Design review of the part built by this model. Coordinates are the model's own, in mm. A direction names the side the tool comes from. Coordinates: 2 decimals unless noted, no trailing zeros. Write each loop counter-clockwise with the first axis right and the second up, starting at its lowest first coordinate (ties: lowest second). Pieces come first, ordered by that corner, then holes. Notation, with made-up numbers: M 58,57.5 L 87,57.5 A26 ccw 87,93.5 Z; hole C 32.5,31 d10. An arc over 180 degrees is marked long. Return JSON: item names as keys, results as strings. Group by question number.
```python
from build123d import *

# Parameters (mm, degrees)
F0_W     = 254
F0_H     = 88.9
F0_R     = 3.81
F0_R_2   = 3.937
F1_DEPTH = 127
F2_T     = -2.54
F3_W     = 2.54
F3_H     = 101.6
F4_DEPTH = 101.6
F5_W     = 254
F5_H     = 12.7
F6_DEPTH = 139.7


with BuildPart() as f1:
    # F0 (on Front) → F1 (new body)
    with BuildSketch(Plane.XZ):
        with Locations((-25.4, -44.45)):
            Rectangle(F0_W, F0_H)
        with Locations((-101.6, -76.2)):
            Circle(F0_R, mode=Mode.SUBTRACT)
        with Locations((25.4, -63.5)):
            Circle(F0_R_2, mode=Mode.SUBTRACT)
    extrude(amount=F1_DEPTH)

    # F2
    f2_openings = [f1.faces().sort_by_distance(p)[0] for p in [
        (-25.35547, 0, -44.344356),
        (-25.4, -63.5, -88.9),
        (101.6, -63.5, -44.45),
    ]]
    offset(amount=F2_T, openings=f2_openings)

    # F3 (on face) → F4 (join)
    with BuildSketch(Plane.XY):
        with Locations((52.07, -50.8)):
            Rectangle(F3_W, F3_H)
    extrude(amount=F4_DEPTH)

    # F5 (on face) → F6 (join)
    with BuildSketch(Plane.XY):
        with Locations((-25.4, -120.65)):
            Rectangle(F5_W, F5_H)
    extrude(amount=F6_DEPTH)

    # F7: F1 across plane


with BuildPart() as f1_1:
    add(f1.part)
    add(f1.part.mirror(Plane.XZ))


solid = f1_1.part
```
Item 1: Add section A-A (z = -76.2). Write out the cut boundary in (x, y), plus the area to 3 significant figures.
Item 2: For pin 1 (6 mm diameter, centred on x = -85, y = 97, fed in from +Z); pin 2 (2 mm diameter, centred on x = 52, y = 71, fed in from +Z); pin 3 (4.5 mm diameter, centred on x = -101.6, z = -76.2, fed in from +Y); pin 4 (8 mm diameter, centred on y = 44.5, z = 67.5, fed in from -X), all flat-tipped, find the tip position at first contact; note any pin that passes through.
Item 3: Machinability: for faces 4 (the flat face through (-27, 114.3, 69)), 5 (the flat face through (53.34, 1, 50)), 6 (the flat face through (-149.86, -2, -46)), which of the approach directions +Z, -Z, +X, -X, +Y, -Y give a long, thin tool a straight path to every point of the face, cutting with its end or side? Answer none if there is none.
Item 4: Add section B-B (x = -101.6). Write out the cut boundary in (y, z), plus the area to 3 significant figures.
Item 5: For line 1 (Z direction, x = -101, y = -46); line 2 (Z direction, x = 25.4, y = -54.5); line 3 (X direction, y = 47, z = -63), list the stretches that pass through material, from the lowest coordinate up.
Item 6: The part is to be moulded in two halves that separate along Y. For faces 1 (the flat face through (-27, -121, 139.7)), 2 (the flat face through (-26, 124.46, -45)), 3 (the flat face through (-27, 127, 24)), say which applies: pulls with the +Y half, pulls with the -Y half, needs draft (parallel to the pull), parting line crosses it, or undercut.
Item 7: Add section C-C (y = 17). Write out the cut boundary in (x, z).
Item 8: Add section D-D (z = 37). Write out the cut boundary in (x, y).
Geometry check:
{
 "1": {"outline": "M -152.4,-127 L -105.41,-127 L -105.41,127 L -152.4,127 Z; M -97.79,-127 L 101.6,-127 L 101.6,-124.46 L -95.25,-124.46 L -95.25,124.46 L 101.6,124.46 L 101.6,127 L -97.79,127 Z; hole M -149.86,-124.46 L -107.95,-124.46 L -107.95,124.46 L -149.86,124.46 Z", "area": "3,150 mm^2"},
 "2": {"pin 1": "z = 0", "pin 2": "z = 101.6", "pin 3": "through", "pin 4": "x = 50.8"},
 "3": {"face 4": "+Z, +X, -X", "face 5": "+Z, +X", "face 6": "-Z"},
 "4": {"outline": "M -127,-88.9 L -124.46,-88.9 L -124.46,-82.55 L 124.46,-82.55 L 124.46,-88.9 L 127,-88.9 L 127,-80.01 L -127,-80.01 Z; M -127,-72.39 L 127,-72.39 L 127,139.7 L 114.3,139.7 L 114.3,0 L -114.3,0 L -114.3,139.7 L -127,139.7 Z; hole M -124.46,-69.85 L 124.46,-69.85 L 124.46,-2.54 L -124.46,-2.54 Z", "area": "5,860 mm^2"},
 "5": {"line 1": "-82.52 to -79.96, -72.44 to -69.88, -2.54 to 0", "line 2": "-69.98 to -67.44, -59.56 to -57.02, -2.54 to 0", "line 3": "-152.4 to -149.86, 18.94 to 21.49, 29.31 to 31.86"},
 "6": {"face 1": "needs draft", "face 2": "undercut", "face 3": "pulls with the +Y half"},
 "7": {"outline": "M -152.4,-88.9 L -149.86,-88.9 L -149.86,-2.54 L 101.6,-2.54 L 101.6,0 L 53.34,0 L 53.34,101.6 L 50.8,101.6 L 50.8,0 L -152.4,0 Z; C -101.6,-76.2 d12.7; C 25.4,-63.5 d12.95; hole C -101.6,-76.2 d7.62; hole C 25.4,-63.5 d7.87"},
 "8": {"outline": "M -152.4,-127 L 101.6,-127 L 101.6,-114.3 L -152.4,-114.3 Z; M -152.4,114.3 L 101.6,114.3 L 101.6,127 L -152.4,127 Z; M 50.8,-101.6 L 53.34,-101.6 L 53.34,101.6 L 50.8,101.6 Z"}
}
